The listing builds one solid part. Answer for the finished solid, in the listing's coordinates (mm). A direction names the side the tool comes from. Give positions to 0.01 mm unless a question says otherwise; leave off trailing zeros. Loops run counter-clockwise (first coordinate to the right, second up) from the corner with the lowest first, then second, coordinate; pieces in that order, holes last. Notation, with made-up numbers: M 80,80.25 L 88,80.25 A29 cw 88,119.25 Z; hole C -34.5,-15.5 d5. An arc over 180 degrees is marked long. Return JSON: item names as keys, results as strings.
from build123d import *

# Parameters (mm, degrees)
F0_R     = 12.5
F0_R_2   = 11
F1_DEPTH = 25
F3_W     = 3.9352367166
F3_H     = 6.3360165805
F4_DEPTH = 4.6
F6_DEPTH = 2


with BuildPart() as f1:
    # F0 (on Top) → F1 (new body)
    with BuildSketch(Plane.XY):
        Circle(F0_R)
        Circle(F0_R_2, mode=Mode.SUBTRACT)
    extrude(amount=-F1_DEPTH)

    # F3 (on Top) → F4 (cut)
    with BuildSketch(Plane.XY):
        with Locations((-0.1754433615, -12.4150682241)):
            Rectangle(F3_W, F3_H)
    extrude(amount=-F4_DEPTH, mode=Mode.SUBTRACT)

    # F5 (on face) → F6 (join)
    with BuildSketch(Plane.XY):
        with BuildLine():
            Line((-2.1430617198, -10.7892208461), (1.7921749968, -10.853023025))
            ThreePointArc((1.7921749968, -10.853023025), (0.1783200847, 10.998554539), (-2.1430617198, -10.7892208461))
        make_face()
    extrude(amount=-F6_DEPTH)


solid = f1.part
(1) Given pin 1 (1.5 mm diameter, centred on x = 5.5, z = -22, fed in from -Y); pin 2 (3 mm diameter, centred on x = 9.5, z = -3.5, fed in from +Y); pin 3 (0.5 mm diameter, centred on x = 0, y = -11.5, fed in from +Z), each flat-ended and moving along its own axis, determine where each tip first touches the part or whether it passes through.
Values follow:
{"pin 1": "y = -11.56", "pin 2": "y = 9.6", "pin 3": "z = -4.6"}
(2) The part is cut by section B-B (y = 0). Determine the outline of the cut face in (x, z).
Values follow:
{"outline": "M -12.5,-25 L -11,-25 L -11,-2 L 11,-2 L 11,-25 L 12.5,-25 L 12.5,0 L -12.5,0 Z"}
(3) The part is cut by section A-A (x = -0.25). Determine the outline of the cut face in (y, z), and give its area (3 significant figures).
Values follow:
{"outline": "M -12.5,-25 L -11,-25 L -11,-4.6 L -12.5,-4.6 Z; M -10.82,-2 L 11,-2 L 11,-25 L 12.5,-25 L 12.5,0 L -10.82,0 Z", "area": "112 mm²"}
(4) A tool of negligible diameter and unlimited length cuts with its end or side. For faces 4 (the flat face through (1.792, -12, -2)), 5 (the cylindrical face through (10.161, -4.213, -13.339)), 6 (the flat face through (0, 0, 0)), from which of +Z, -Z, +X, -X, +Y, -Y can it reach the whole face along a straight path? Write none if from no direction.
Values follow:
{"face 4": "+Z, -Y", "face 5": "-Z", "face 6": "+Z, +X, -X, +Y, -Y"}
(5) Straight lines are drawn through the part: line 1 along Y through (x, z) = (0, -15); line 2 along Z through (x, y) = (10.75, -2). For each, find the intervals that lie inside material, in ascending order.
Values follow:
{"line 1": "-12.5 to -11, 11 to 12.5", "line 2": "-2 to 0"}
(6) Determine the mould class of faces 1 (the flat face through (-2.143, -12, -2)), 2 (the cylindrical face through (11.923, 3.755, -12.325)), 3 (the flat face through (5, -10, -25)) for opening direction X: released by +X, released by -X, zero draft, split by the parting line, or undercut.
Values follow:
{"face 1": "undercut", "face 2": "split by the parting line", "face 3": "zero draft"}
(7) The part is cut by section C-C (z = -15.25). Determine the outline of the cut face in (x, y), and give its area (3 significant figures).
Values follow:
{"outline": "C 0,0 d25; hole C 0,0 d22", "area": "111 mm²"}
(8) The part is cut by section D-D (x = -6). Determine the outline of the cut face in (y, z), and give its area (3 significant figures).
Values follow:
{"outline": "M -10.97,-25 L -9.22,-25 L -9.22,-2 L 9.22,-2 L 9.22,-25 L 10.97,-25 L 10.97,0 L -10.97,0 Z", "area": "124 mm²"}
